Read the model definition and answer for the solid it produces. Units are mm, in the model's axes. Face numbers are marked on the shaded views. A direction names the side the tool comes from. Coordinates: 2 decimals unless noted, no trailing zeros. Write each loop counter-clockwise with the first axis right and the second up, starting at its lowest first coordinate (ties: lowest second). Pieces come first, ordered by that corner, then holes. Notation, with made-up numbers: (53.5, -29.75) - (95.5, -29.75) arc R17 cw to (95.5, -5.75) - close; hole circle Ø7 at (6, -40). An arc over 180 degrees is marked (long way). Use a Markdown table: item, result.
from build123d import *
from build123d import SkipClean  # not in build123d's __all__

# Parameters (mm, degrees)
F0_R          = 6.5
F1_DEPTH      = 1
F3_DEPTH      = 11
F7_R          = 1.375
F8_DEPTH      = 12
F9_W          = 46.4800073215
F9_H          = 2
F10_DEPTH     = 12
F11_T4_DEPTH  = 10.4788869849
F11_S5_R      = 1.375
F11_T6_DEPTH  = 7
F11_S7_R      = 6.5
F11_T8_DEPTH  = 7
F11_T12_DEPTH = 10.4788869849
F11_S13_R     = 6.5
F11_T14_DEPTH = 7
F11_S15_R     = 1.375
F11_T16_DEPTH = 7
F11_T20_DEPTH = 10.4788869849
F11_S21_R     = 1.375
F11_T22_DEPTH = 7
F11_S23_R     = 6.5
F11_T24_DEPTH = 7
F11_T28_DEPTH = 10.4788869849
F11_S29_R     = 1.375
F11_T30_DEPTH = 7
F11_S31_R     = 6.5
F11_T32_DEPTH = 7
F11_T36_DEPTH = 17.3693168769
F11_S37_R     = 6.5
F11_T38_DEPTH = 10
F11_T42_DEPTH = 17.3693168769
F11_S43_R     = 6.5
F11_T44_DEPTH = 10


# Not quite as in the source:
# - a fillet or chamfer that OpenCascade refuses, or shapes differently, is made with other operations: its cross-section is extruded or revolved along the edge and cut away or added
# - after a boolean that leaves OpenCascade's solid faulty, fix() repairs it


with BuildPart() as f1:
    # F0 (on Top) → F1 (new body, symmetric)
    with BuildSketch(Plane.XY):
        Circle(F0_R)
    extrude(amount=F1_DEPTH, both=True)

    # F2 (on face) → F3 (join)
    with BuildSketch(Plane.XY.offset(1)):
        with BuildLine():
            ThreePointArc((6.5, 0), (6.4206806434, 1.0123537302), (6.1846584384, 2))
            Line((6.1846584384, 2), (-6.1846584384, 2))
            ThreePointArc((-6.1846584384, 2), (-6.5, 0), (-6.1846584384, -2))
            Line((-6.1846584384, -2), (6.1846584384, -2))
            ThreePointArc((6.1846584384, -2), (6.4206806434, -1.0123537302), (6.5, 0))
        make_face()
    with SkipClean():  # cleaning this boolean's faces spoils the solid; the shape is the same uncleaned
        extrude(amount=F3_DEPTH)

    # F5 (on offset) → F6 section 0
    with BuildSketch(Plane.XY.offset(4)):
        with BuildLine():
            ThreePointArc((5.7662812973, -3), (6.5, 0), (5.7662812973, 3))
            Line((5.7662812973, 3), (-5.7662812973, 3))
            ThreePointArc((-5.7662812973, 3), (-6.5, 0), (-5.7662812973, -3))
            Line((-5.7662812973, -3), (5.7662812973, -3))
        make_face()
    # F3_face (on face) → F6 section 1
    with BuildSketch(Plane.XY.offset(12)):
        with BuildLine():
            ThreePointArc((6.1846584384, -2), (6.5, 0), (6.1846584384, 2))
            Line((6.1846584384, 2), (-6.1846584384, 2))
            ThreePointArc((-6.1846584384, 2), (-6.5, 0), (-6.1846584384, -2))
            Line((-6.1846584384, -2), (6.1846584384, -2))
        make_face()
    loft()

    add(f1.part.fix(), mode=Mode.REPLACE)

    # F7 (on face) → F8 (cut)
    with BuildSketch(Plane(origin=(0, 0, -1), x_dir=(1, 0, 0), z_dir=(0, 0, -1))):
        Circle(F7_R)
    extrude(amount=-F8_DEPTH, mode=Mode.SUBTRACT)

    # F9 (on face) → F10 (cut)
    with BuildSketch(Plane(origin=(0, 0, -1), x_dir=(1, 0, 0), z_dir=(0, 0, -1))):
        Rectangle(F9_W, F9_H)
    extrude(amount=-F10_DEPTH, mode=Mode.SUBTRACT)

    # F11: fillet of radius 1 on 8 edges, made by hand


with BuildPart() as f11_tool2:
    # F11_s3 → F11_t4 (new body)
    with BuildSketch(Plane.YZ.offset(-8.9226162893)):
        with BuildLine():
            ThreePointArc((0, 11), (0.7071067812, 10.7071067812), (1, 10))
            Line((1, 10), (1, 11))
            Line((1, 11), (0, 11))
        make_face()
    extrude(amount=F11_T4_DEPTH)

    # F11_s5 → F11_t6 (cut, symmetric)
    with BuildSketch(Plane.XY.offset(10.5)):
        Circle(F11_S5_R)
    extrude(amount=F11_T6_DEPTH, both=True, mode=Mode.SUBTRACT)

    # F11_s7 → F11_t8 (intersect, symmetric)
    with BuildSketch(Plane.XY.offset(10.5)):
        Circle(F11_S7_R)
    extrude(amount=F11_T8_DEPTH, both=True, mode=Mode.INTERSECT)


with BuildPart() as f1_1:
    add(f1.part, clean=False)

    # F11_t1: union F11_tool2
    add(f11_tool2.part)


with BuildPart() as f11_tool10:
    # F11_s11 → F11_t12 (new body)
    with BuildSketch(Plane.YZ.offset(-1.5562706956)):
        with BuildLine():
            ThreePointArc((1, 10), (0.7071067812, 10.7071067812), (0, 11))
            Line((0, 11), (1, 11))
            Line((1, 11), (1, 10))
        make_face()
    extrude(amount=F11_T12_DEPTH)

    # F11_s13 → F11_t14 (intersect, symmetric)
    with BuildSketch(Plane.XY.offset(10.5)):
        Circle(F11_S13_R)
    extrude(amount=F11_T14_DEPTH, both=True, mode=Mode.INTERSECT)

    # F11_s15 → F11_t16 (cut, symmetric)
    with BuildSketch(Plane.XY.offset(10.5)):
        Circle(F11_S15_R)
    extrude(amount=F11_T16_DEPTH, both=True, mode=Mode.SUBTRACT)


with BuildPart() as f1_2:
    add(f1_1.part, clean=False)

    # F11_t9: union F11_tool10
    add(f11_tool10.part)


with BuildPart() as f11_tool18:
    # F11_s19 → F11_t20 (new body)
    with BuildSketch(Plane.YZ.offset(8.9226162893)):
        with BuildLine():
            ThreePointArc((-1, 10), (-0.7071067812, 10.7071067812), (0, 11))
            Line((0, 11), (-1, 11))
            Line((-1, 11), (-1, 10))
        make_face()
    extrude(amount=-F11_T20_DEPTH)

    # F11_s21 → F11_t22 (cut, symmetric)
    with BuildSketch(Plane.XY.offset(10.5)):
        Circle(F11_S21_R)
    extrude(amount=F11_T22_DEPTH, both=True, mode=Mode.SUBTRACT)

    # F11_s23 → F11_t24 (intersect, symmetric)
    with BuildSketch(Plane.XY.offset(10.5)):
        Circle(F11_S23_R)
    extrude(amount=F11_T24_DEPTH, both=True, mode=Mode.INTERSECT)


with BuildPart() as f1_3:
    add(f1_2.part, clean=False)

    # F11_t17: union F11_tool18
    add(f11_tool18.part)


with BuildPart() as f11_tool26:
    # F11_s27 → F11_t28 (new body)
    with BuildSketch(Plane.YZ.offset(1.5562706956)):
        with BuildLine():
            ThreePointArc((0, 11), (-0.7071067812, 10.7071067812), (-1, 10))
            Line((-1, 10), (-1, 11))
            Line((-1, 11), (0, 11))
        make_face()
    extrude(amount=-F11_T28_DEPTH)

    # F11_s29 → F11_t30 (cut, symmetric)
    with BuildSketch(Plane.XY.offset(10.5)):
        Circle(F11_S29_R)
    extrude(amount=F11_T30_DEPTH, both=True, mode=Mode.SUBTRACT)

    # F11_s31 → F11_t32 (intersect, symmetric)
    with BuildSketch(Plane.XY.offset(10.5)):
        Circle(F11_S31_R)
    extrude(amount=F11_T32_DEPTH, both=True, mode=Mode.INTERSECT)


with BuildPart() as f1_4:
    add(f1_3.part, clean=False)

    # F11_t25: union F11_tool26
    add(f11_tool26.part)


with BuildPart() as f11_tool34:
    # F11_s35 → F11_t36 (new body)
    with BuildSketch(Plane.YZ.offset(8.6846584384)):
        with BuildLine():
            ThreePointArc((3, 1), (2.2928932188, 1.2928932188), (2, 2))
            Line((2, 2), (2, 1))
            Line((2, 1), (3, 1))
        make_face()
    extrude(amount=-F11_T36_DEPTH)

    # F11_s37 → F11_t38 (intersect, symmetric)
    with BuildSketch(Plane.XY.offset(1.5)):
        Circle(F11_S37_R)
    extrude(amount=F11_T38_DEPTH, both=True, mode=Mode.INTERSECT)


with BuildPart() as f1_5:
    add(f1_4.part, clean=False)

    # F11_t33: union F11_tool34
    add(f11_tool34.part)


with BuildPart() as f11_tool40:
    # F11_s41 → F11_t42 (new body)
    with BuildSketch(Plane.YZ.offset(-8.6846584384)):
        with BuildLine():
            ThreePointArc((-2, 2), (-2.2928932188, 1.2928932188), (-3, 1))
            Line((-3, 1), (-2, 1))
            Line((-2, 1), (-2, 2))
        make_face()
    extrude(amount=F11_T42_DEPTH)

    # F11_s43 → F11_t44 (intersect, symmetric)
    with BuildSketch(Plane.XY.offset(1.5)):
        Circle(F11_S43_R)
    extrude(amount=F11_T44_DEPTH, both=True, mode=Mode.INTERSECT)


with BuildPart() as f1_6:
    add(f1_5.part, clean=False)

    # F11_t39: union F11_tool40
    add(f11_tool40.part)


solid = f1_6.part
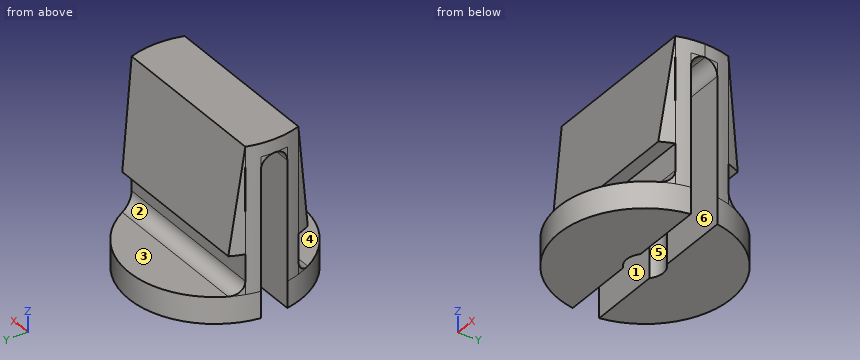
(1) Each of these flat-tipped pins is pushed along its axis until it touches: P1, Ø6, axis at x = 3.5, z = 6, coming from the -Y side; P2, Ø2.5, axis at x = 3.5, z = 6, coming from the +Y side; P3, Ø1.6, axis at x = -0.5, z = 3, coming from the -Y side. Where does it stop, or does it pass through?
Report:
| item | result |
|---|---|
| P1 | stops at y = -3 |
| P2 | stops at y = 2.91 |
| P3 | stops at y = -2 |
(2) A cutting plane is placed at A-A, the plane z = 1.5. Write down the section's boundary in (x, y) (3 decimals).
Report:
| item | result |
|---|---|
| outline | (-6.423, -1) arc R6.5 ccw to (-6.14, -2.134) - (6.14, -2.134) arc R6.5 ccw to (6.423, -1) - (0.944, -1) arc R1.375 cw to (-0.944, -1) - close; (-6.423, 1) - (-0.944, 1) arc R1.375 cw to (0.944, 1) - (6.423, 1) arc R6.5 ccw to (6.14, 2.134) - (-6.14, 2.134) arc R6.5 ccw to start |
(3) The mould has two halves that part along Y. Classify the marked faces 1, 2 and 3: pulls with the +Y half, pulls with the -Y half, needs draft (parallel to the pull), parting line crosses it, or undercut.
Report:
| item | result |
|---|---|
| face 1 | undercut |
| face 2 | pulls with the +Y half |
| face 3 | needs draft |
(4) For the marked faces 4, 5 and 6, determine the directions among +Z, -Z, +X, -X, +Y, -Y from which every point of the face is accessible in a straight line to the end or side of a thin tool.
Report:
| item | result |
|---|---|
| face 4 | +Z, +X, -X, -Y |
| face 5 | -Z |
| face 6 | -Z, +X, -X |
(5) Straight lines are drawn through the part: L1, parallel to Y at x = -5.5, z = 2.5; L2, parallel to Y at x = 1, z = 10.75; L3, parallel to Z at x = -1.5, y = 4.5. For each, find the intervals that lie inside material, in ascending order.
Report:
| item | result |
|---|---|
| L1 | y = -2 to -1, 1 to 2 |
| L2 | y = -2.16 to -0.94, 0.94 to 2.16 |
| L3 | z = -1 to 1 |
